```python
from build123d import *

# Parameters (mm, degrees)
ESQUISSE1_R      = 1.5
EXTRUSION1_DEPTH = 2


with BuildPart() as part:
    # Esquisse1 → Extrusion1 (new body)
    with BuildSketch(Plane.XY):
        Polygon((5.264207965, 14.044526316), (65.264207965, 14.044526316), (65.264207965, -45.955473684), (52.264207965, -45.955473684), (52.264207965, -57.955473684), (18.264207965, -57.955473684), (18.264207965, -45.955473684), (5.264207965, -45.955473684), align=None)
        with Locations((57.764207965, 1.544526316)):
            Circle(ESQUISSE1_R, mode=Mode.SUBTRACT)
        with Locations((57.764207965, -6.455473684)):
            Circle(ESQUISSE1_R, mode=Mode.SUBTRACT)
        with Locations((12.764207965, -33.455473684)):
            Circle(ESQUISSE1_R, mode=Mode.SUBTRACT)
        with Locations((12.764207965, -25.455473684)):
            Circle(ESQUISSE1_R, mode=Mode.SUBTRACT)
        with Locations((40.264207965, -43.955473684)):
            Circle(ESQUISSE1_R, mode=Mode.SUBTRACT)
        with Locations((30.264207965, -43.955473684)):
            Circle(ESQUISSE1_R, mode=Mode.SUBTRACT)
        with Locations((49.764207965, -17.955473684)):
            Circle(ESQUISSE1_R, mode=Mode.SUBTRACT)
        with Locations((59.764207965, -17.955473684)):
            Circle(ESQUISSE1_R, mode=Mode.SUBTRACT)
        with Locations((31.764207965, 7.044526316)):
            Circle(ESQUISSE1_R, mode=Mode.SUBTRACT)
        with Locations((38.764207965, 7.044526316)):
            Circle(ESQUISSE1_R, mode=Mode.SUBTRACT)
        with Locations((22.264207965, 3.544526316)):
            Circle(ESQUISSE1_R, mode=Mode.SUBTRACT)
        with Locations((48.264207965, 3.544526316)):
            Circle(ESQUISSE1_R, mode=Mode.SUBTRACT)
        with Locations((20.764207965, -13.955473684)):
            Circle(ESQUISSE1_R, mode=Mode.SUBTRACT)
        with Locations((10.764207965, -13.955473684)):
            Circle(ESQUISSE1_R, mode=Mode.SUBTRACT)
        with Locations((22.264207965, -51.955473684)):
            Circle(ESQUISSE1_R, mode=Mode.SUBTRACT)
        with Locations((48.264207965, -51.955473684)):
            Circle(ESQUISSE1_R, mode=Mode.SUBTRACT)
    extrude(amount=EXTRUSION1_DEPTH)


solid = part.part
```
Build history of the part. All positions in model axes, mm. A direction names the side the tool comes from. Coordinates: 2 decimals unless noted, no trailing zeros. Order: outer loops, then holes, each group sorted by start corner. A loop starts at its lowest first (then second) coordinate and runs counter-clockwise, first axis right, second up. Notation, with made-up numbers: (-8, 62) -> (40, 62) arc R13 cw to (40, 75) -> close; hole circle Ø3 at (30.5, 14). An arc over 180 degrees is marked (long way). Answer in a Markdown table with one row per item. Add a question column.
Q1. Which spindle directions (+Z, -Z, +X, -X, +Y, -Y) get a long thin tool onto all of the face, cutting with end or side? Do faces 4 (the face through (18.264, -52, 1)), 5 (the face through (59, -45.955, 1)), 6 (the face through (12.57, -31.97, 0.99)). Say none if no direction does.
Q2. Drop flat-ended pins along their axis: pin 1 (4 mm diameter, centred on x = 57.76, y = 1.54, fed in from -Z); pin 2 (2.5 mm diameter, centred on x = 59.76, y = -17.96, fed in from +Z); pin 3 (0.6 mm diameter, centred on x = 11, z = 1.5, fed in from -Y); pin 4 (0.6 mm diameter, centred on y = -53.5, z = 0.5, fed in from +X). Give the stop position or say it passes through.
Q3. Band-saw the part on B-B, the plane z = 1.5. Give the number of separate pieces and of enclosed holes in the cut face, then the cut area to 3 significant figures.
Q4. Band-saw the part on C-C, the plane x = 53.5. List the corners of the cut face in (y, z), then the cut area to 3 significant figures.
Q5. Wall check: line 1 along X through (y, z) = (-18, 0.4); line 2 along Y through (x, z) = (49, 1.05); line 3 along Y through (x, z) = (50, 1.8). Give the ranges that are in metal, low to high. Write a range as [from, to].
Q6. Mould opens along Y. For faces 1 (the face through (30.266, 7.11, 0.986)), 2 (the face through (36, -21, 0)), 3 (the face through (36, -57.955, 1)) say: +Y half, -Y half, draft (parallel to the pull), parting line (faces both ways), or undercut.
Q7. Band-saw the part on A-A, the plane x = 60.5. List the corners of the cut face in (y, z), then the cut area to 3 significant figures.
Answers follow:
| question | item | result |
|---|---|---|
| 1 | face 4 | +Z, -Z, -X, -Y |
| 1 | face 5 | +Z, -Z, +X, -Y |
| 1 | face 6 | +Z, -Z |
| 2 | pin 1 | z = 0 |
| 2 | pin 2 | through |
| 2 | pin 3 | y = -45.96 |
| 2 | pin 4 | x = 52.26 |
| 3 | separate pieces | 1 |
| 3 | enclosed holes | 16 |
| 3 | area | 3,890 mm^2 |
| 4 | outline | (-45.96, 0) -> (14.04, 0) -> (14.04, 2) -> (-45.96, 2) -> close |
| 4 | area | 120 mm^2 |
| 5 | line 1 | [5.26, 48.26], [51.26, 58.26], [61.26, 65.26] |
| 5 | line 2 | [-57.96, -53.26], [-50.65, -19.25], [-16.66, 2.24], [4.85, 14.04] |
| 5 | line 3 | [-57.96, -19.44], [-16.47, 14.04] |
| 6 | face 1 | undercut |
| 6 | face 2 | draft |
| 6 | face 3 | -Y half |
| 7 | outline | (-45.96, 0) -> (-19.26, 0) -> (-19.26, 2) -> (-45.96, 2) -> close; (-16.65, 0) -> (14.04, 0) -> (14.04, 2) -> (-16.65, 2) -> close |
| 7 | area | 115 mm^2 |
